from build123d import *

# Parameters (mm, degrees)
BOSS_EXTRUDE1_OUTLINE_R = 1.3462
BOSS_EXTRUDE1_DEPTH     = 3.048
SKETCH14_W              = 2.2754
SKETCH14_H              = 2.1513
CUT_EXTRUDE2_DEPTH      = 430.898988368
SKETCH15_W              = 16.8402
SKETCH15_H              = 14.1197
SKETCH15_H_2            = 15.4101
CUT_EXTRUDE3_DEPTH      = 430.898988368
SKETCH16_R              = 1.524
CUT_EXTRUDE4_DEPTH      = 430.898988368
SKETCH17_W              = 13.7159
SKETCH17_H              = 5.7149
SKETCH17_W_2            = 4.1917
SKETCH17_H_2            = 7.175
CUT_EXTRUDE5_DEPTH      = 430.898988368
SKETCH18_W              = 1.778
SKETCH18_H              = 5.3847
BOSS_EXTRUDE9_DEPTH     = 3.048


# Read off the part's stored shape, not the designer's step: Boss-Extrude1
with BuildPart() as part:
    # Boss-Extrude1 outline → Boss-Extrude1 (new body)
    with BuildSketch(Plane.XY):
        with BuildLine():
            ThreePointArc((-397.247125, 154.7804), (-399.946077222, 153.659592612), (-401.0571, 150.956597849))
            Line((-401.0571, 150.956597849), (-401.0571, 148.341))
            Line((-401.0571, 148.341), (-388.8032, 148.341))
            Line((-388.8032, 148.341), (-388.8032, 149.5347))
            Line((-388.8032, 149.5347), (-375.7222, 149.5347))
            Line((-375.7222, 149.5347), (-375.7222, 144.15))
            Line((-375.7222, 144.15), (-380.1672, 144.15))
            Line((-380.1672, 144.15), (-380.1672, 132.9309))
            Line((-380.1672, 132.9309), (-396.8172, 132.9309))
            Line((-396.8172, 132.9309), (-396.8172, 129.2706))
            Line((-396.8172, 129.2706), (-380.1672, 129.2706))
            Line((-380.1672, 129.2706), (-380.1672, 120.8224))
            Line((-380.1672, 120.8224), (-375.3812, 120.8224))
            Line((-375.3812, 120.8224), (-375.3812, 118.2824))
            Line((-375.3812, 118.2824), (-375.1272, 118.2824))
            Line((-375.1272, 118.2824), (-375.1272, 115.1509))
            Line((-375.1272, 115.1509), (-396.8172, 115.1509))
            Line((-396.8172, 115.1509), (-396.8172, 111.6447))
            Line((-396.8172, 111.6447), (-373.7775, 111.6447))
            Line((-373.7775, 111.6447), (-373.7775, 99.7089))
            Line((-373.7775, 99.7089), (-375.4172, 99.7089))
            Line((-375.4172, 99.7089), (-375.4172, 95.6449))
            Line((-375.4172, 95.6449), (-401.0571, 95.6449))
            Line((-401.0571, 95.6449), (-401.0571, 91.659304166))
            ThreePointArc((-401.0571, 91.659304166), (-399.951018769, 88.947400452), (-397.2472, 87.8217))
            Line((-397.2472, 87.8217), (-378.5565, 87.8217))
            Line((-378.5565, 87.8217), (-368.3165, 91.1883))
            Line((-368.3165, 91.1883), (-368.3165, 99.7089))
            Line((-368.3165, 99.7089), (-371.8725, 99.7089))
            Line((-371.8725, 99.7089), (-371.8725, 103.0109))
            Line((-371.8725, 103.0109), (-370.6025, 103.0109))
            Line((-370.6025, 103.0109), (-370.6025, 113.7612))
            Line((-370.6025, 113.7612), (-356.8152, 113.7612))
            Line((-356.8152, 113.7612), (-356.8152, 115.9125))
            Line((-356.8152, 115.9125), (-353.6872, 115.9125))
            Line((-353.6872, 115.9125), (-353.6872, 93.3059))
            Line((-353.6872, 93.3059), (-360.5003, 93.3059))
            Line((-360.5003, 93.3059), (-360.5003, 91.1883))
            Line((-360.5003, 91.1883), (-350.7686, 91.1883))
            Line((-350.7686, 91.1883), (-350.7686, 98.2843))
            Line((-350.7686, 98.2843), (-352.4372, 98.2843))
            Line((-352.4372, 98.2843), (-352.4372, 102.1451))
            Line((-352.4372, 102.1451), (-350.7686, 102.1451))
            Line((-350.7686, 102.1451), (-350.7686, 108.2665))
            Line((-350.7686, 108.2665), (-333.6613, 108.2665))
            Line((-333.6613, 108.2665), (-333.6613, 113.4801))
            Line((-333.6613, 113.4801), (-324.6295, 113.4801))
            Line((-324.6295, 113.4801), (-324.6295, 103.9551))
            Line((-324.6295, 103.9551), (-320.8233, 103.9551))
            Line((-320.8233, 103.9551), (-320.8233, 102.0978))
            Line((-320.8233, 102.0978), (-319.8913, 102.0978))
            Line((-319.8913, 102.0978), (-319.8913, 99.5578))
            Line((-319.8913, 99.5578), (-322.0933, 99.5578))
            Line((-322.0933, 99.5578), (-322.0933, 100.5738))
            Line((-322.0933, 100.5738), (-327.8337, 100.5738))
            Line((-327.8337, 100.5738), (-327.8337, 94.1717))
            Line((-327.8337, 94.1717), (-334.5393, 94.1717))
            Line((-334.5393, 94.1717), (-334.5393, 91.1883))
            Line((-334.5393, 91.1883), (-324.8873, 91.1883))
            Line((-324.8873, 91.1883), (-324.8873, 98.5911))
            Line((-324.8873, 98.5911), (-315.9973, 98.5911))
            Line((-315.9973, 98.5911), (-315.9973, 91.1883))
            Line((-315.9973, 91.1883), (-305.7573, 87.8217))
            ThreePointArc((-305.7573, 87.8217), (-303.063223164, 88.937623164), (-301.9473, 91.6317))
            Line((-301.9473, 91.6317), (-301.9473, 150.9704))
            ThreePointArc((-301.9473, 150.9704), (-303.063223164, 153.664476836), (-305.7573, 154.7804))
            Line((-305.7573, 154.7804), (-397.247125, 154.7804))
        make_face()
        with Locations((-397.2472, 91.6317)):
            Circle(BOSS_EXTRUDE1_OUTLINE_R, mode=Mode.SUBTRACT)
        with Locations((-305.7573, 91.6317)):
            Circle(BOSS_EXTRUDE1_OUTLINE_R, mode=Mode.SUBTRACT)
        Polygon((-322.5975, 105.3521), (-322.5975, 113.4801), (-316.4253, 113.4801), (-316.4253, 134.0739), (-310.8373, 134.0739), (-310.8373, 100.5738), (-317.7753, 100.5738), (-317.7753, 103.0869), (-319.8913, 103.0869), (-319.8913, 105.3521), align=None, mode=Mode.SUBTRACT)
        Polygon((-372.7142, 122.6512), (-372.7142, 132.9309), (-377.6672, 132.9309), (-377.6672, 140.2451), (-357.2832, 140.2451), (-357.2832, 124.1751), (-352.2032, 124.1751), (-352.2032, 118.8412), (-373.2222, 118.8412), (-373.2222, 122.6512), align=None, mode=Mode.SUBTRACT)
        with Locations((-397.247125, 150.9704)):
            Circle(BOSS_EXTRUDE1_OUTLINE_R, mode=Mode.SUBTRACT)
        Polygon((-335.9473, 116.6297), (-335.9473, 114.6425), (-350.1712, 114.6425), (-350.1712, 134.8668), (-318.2033, 134.8668), (-318.2033, 116.6297), align=None, mode=Mode.SUBTRACT)
        Polygon((-310.8374, 136.3599), (-316.4253, 136.3599), (-316.4253, 136.6448), (-340.5193, 136.6448), (-340.5193, 142.3597), (-371.5305, 142.3597), (-371.5305, 150.1697), (-310.8373, 150.1697), align=None, mode=Mode.SUBTRACT)
        with Locations((-305.7573, 150.9704)):
            Circle(BOSS_EXTRUDE1_OUTLINE_R, mode=Mode.SUBTRACT)
    extrude(amount=BOSS_EXTRUDE1_DEPTH)

    # Sketch14 → Cut-Extrude2 (cut, through all)
    with BuildSketch(Plane(origin=(0, 0, 0), x_dir=(-1, 0, 0), z_dir=(0, 0, -1))):
        with Locations((357.9529, 114.83685)):
            Rectangle(SKETCH14_W, SKETCH14_H)
    extrude(amount=-CUT_EXTRUDE2_DEPTH, mode=Mode.SUBTRACT)

    # Sketch15 → Cut-Extrude3 (cut, through all)
    with BuildSketch(Plane(origin=(0, 0, 0), x_dir=(-1, 0, 0), z_dir=(0, 0, -1))):
        with Locations((388.3971, 122.21075)):
            Rectangle(SKETCH15_W, SKETCH15_H)
        with Locations((388.3971, 140.63595)):
            Rectangle(SKETCH15_W, SKETCH15_H_2)
    extrude(amount=-CUT_EXTRUDE3_DEPTH, mode=Mode.SUBTRACT)

    # Sketch16 → Cut-Extrude4 (cut, through all)
    with BuildSketch(Plane.XY.offset(3.048)):
        with Locations((-397.247125, 150.9704)):
            Circle(SKETCH16_R)
        with Locations((-305.7573, 150.9704)):
            Circle(SKETCH16_R)
        with Locations((-305.7573, 91.6317)):
            Circle(SKETCH16_R)
        with Locations((-397.2472, 91.6317)):
            Circle(SKETCH16_R)
    extrude(amount=-CUT_EXTRUDE4_DEPTH, mode=Mode.SUBTRACT)

    # Sketch17 → Cut-Extrude5 (cut, through all)
    with BuildSketch(Plane(origin=(0, 0, 0), x_dir=(-1, 0, 0), z_dir=(0, 0, -1))):
        with Locations((347.37725, 139.50225)):
            Rectangle(SKETCH17_W, SKETCH17_H)
        with Locations((373.62635, 145.9472)):
            Rectangle(SKETCH17_W_2, SKETCH17_H_2)
    extrude(amount=-CUT_EXTRUDE5_DEPTH, mode=Mode.SUBTRACT)

    # Sketch18 → Boss-Extrude9 (add)
    with BuildSketch(Plane(origin=(0, 0, 0), x_dir=(-1, 0, 0), z_dir=(0, 0, -1))):
        with Locations((376.6112, 146.84235)):
            Rectangle(SKETCH18_W, SKETCH18_H)
    extrude(amount=-BOSS_EXTRUDE9_DEPTH)


solid = part.part
Design review of the part built by this model. Coordinates are the model's own, in mm. A direction names the side the tool comes from. Round coordinates to 2 decimals unless told otherwise and drop trailing zeros. Write each loop counter-clockwise with the first axis right and the second up, starting at its lowest first coordinate (ties: lowest second). Pieces come first, ordered by that corner, then holes. Notation, with made-up numbers: (-26, -38) - (-14, -38) arc R22 cw to (-14, -13) - close; hole circle Ø6 at (27.5, 77.25). An arc over 180 degrees is marked (long way). Return JSON: item names as keys, results as strings. Group by question number.
Item 1: We need section D-D on z = 1.75. Give the number of separate pieces and of enclosed holes in the cut face, and give its area (3 significant figures).
Item 2: Insertion check: P1, Ø0.9, axis at x = -378.5, z = 2, coming from the -Y side; P2, Ø0.7, axis at x = -320.5, z = 1.5, coming from the -Y side; P3, Ø1.5, axis at y = 103, z = 1, coming from the -X side. Each pin has a flat end and moves straight along its axis. Give the tip position at first contact, or say it passes through.
Item 3: For probe 1 along X at (y, z) = (107.5, 2.3); probe 2 along X at (y, z) = (101, 0.3); probe 3 along Y at (x, z) = (-380.5, 0.2), list the stretches that pass through material, from the lowest coordinate up. Write a range as [from, to].
Item 4: We need section B-B on x = -382. Write out the cut boundary in (y, z).
Item 5: We need section C-C on y = 107. Write out the cut boundary in (x, z).
Item 6: We need section A-A on x = -342.5. Write out the cut boundary in (y, z), and give its area (3 significant figures).
Item 7: Machinability: for faces 5 (the face through (-375.722, 146, 2)), 6 (the face through (-375.417, 98, 2)), which of the approach directions +Z, -Z, +X, -X, +Y, -Y give a long, thin tool a straight path to every point of the face, cutting with its end or side? Answer none if there is none.
Item 8: The part is to be moulded in two halves that separate along Y. For faces 1 (the face through (-315.997, 95, 2)), 2 (the face through (-321, 105.352, 2)), 3 (the face through (-371.872, 101, 2)), 4 (the face through (-330, 91.188, 2)), say which applies: pulls with the +Y half, pulls with the -Y half, needs draft (parallel to the pull), parting line crosses it, or undercut.
Model answer:
{
 "1": {"separate pieces": "1", "enclosed holes": "8", "area": "2,350 mm²"},
 "2": {"P1": "stops at y = 87.82", "P2": "stops at y = 98.59", "P3": "stops at x = -373.78"},
 "3": {"probe 1": "x = [-373.78, -370.6], [-353.69, -350.77], [-324.63, -322.6], [-310.84, -301.95]", "probe 2": "x = [-373.78, -371.87], [-353.69, -352.44], [-319.89, -317.78], [-310.84, -301.95]", "probe 3": "y = [87.82, 95.64], [111.64, 115.15], [129.27, 132.93], [149.53, 154.78]"},
 "4": {"outline": "(87.82, 0) - (95.64, 0) - (95.64, 3.05) - (87.82, 3.05) - close; (111.64, 0) - (115.15, 0) - (115.15, 3.05) - (111.64, 3.05) - close; (129.27, 0) - (132.93, 0) - (132.93, 3.05) - (129.27, 3.05) - close; (149.53, 0) - (154.78, 0) - (154.78, 3.05) - (149.53, 3.05) - close"},
 "5": {"outline": "(-373.78, 0) - (-370.6, 0) - (-370.6, 3.05) - (-373.78, 3.05) - close; (-353.69, 0) - (-350.77, 0) - (-350.77, 3.05) - (-353.69, 3.05) - close; (-324.63, 0) - (-322.6, 0) - (-322.6, 3.05) - (-324.63, 3.05) - close; (-310.84, 0) - (-301.95, 0) - (-301.95, 3.05) - (-310.84, 3.05) - close"},
 "6": {"outline": "(108.27, 0) - (114.64, 0) - (114.64, 3.05) - (108.27, 3.05) - close; (134.87, 0) - (136.64, 0) - (136.64, 3.05) - (134.87, 3.05) - close; (150.17, 0) - (154.78, 0) - (154.78, 3.05) - (150.17, 3.05) - close", "area": "38.9 mm²"},
 "7": {"face 5": "+Z, -Z", "face 6": "+Z, -Z, -X"},
 "8": {"face 1": "needs draft", "face 2": "undercut", "face 3": "undercut", "face 4": "pulls with the -Y half"}
}
